```python
from build123d import *

# Parameters (mm, degrees)
ESQUISSE1_R        = 2.5
BOSS_EXTRU_2_DEPTH = 5
CONG_2_R           = 2


with BuildPart() as part:
    # Esquisse1 → Boss.-Extru.2 (new body)
    with BuildSketch(Plane.XY):
        Polygon((-39.751873238, 27.403100775), (30.248126762, 27.403100775), (30.248126762, -27.596899225), (14.016967887, -27.596899225), (-39.751873238, 24.689922481), align=None)
        with Locations((22.936263184, 20.04525616)):
            Circle(ESQUISSE1_R, mode=Mode.SUBTRACT)
        with Locations((22.936263184, -19.519610844)):
            Circle(ESQUISSE1_R, mode=Mode.SUBTRACT)
    extrude(amount=BOSS_EXTRU_2_DEPTH)

    # Congé2
    cong_2_edges = [part.edges().sort_by_distance(p)[0] for p in [
        (-39.751873238, 24.689922481, 2.5),
    ]]
    fillet(cong_2_edges, radius=CONG_2_R)


solid = part.part
```
Geometry: final body of the model. Coordinates: model frame, mm. Give positions to 0.01 mm unless a question says otherwise; leave off trailing zeros. Loops run counter-clockwise (first coordinate to the right, second up) from the corner with the lowest first, then second, coordinate; pieces in that order, holes last. Notation, with made-up numbers: (-25, 39) -> (11, 39) arc R21 cw to (11, 45) -> close; hole circle Ø3 at (35, 27.5). An arc over 180 degrees is marked (long way). Use CSV: the item, a comma, the result in double quotes.
(1) Pull-direction query (X, two-part tool) for faces 1 (the face through (21.09, 21.73, 2.46)), 2 (the face through (-12.2, -2.1, 2.5)), 3 (the face through (30.248, 0, 2)); classes: released by +X, released by -X, zero draft, split by the parting line, or undercut.
From the geometry:
face 1,"undercut"
face 2,"released by -X"
face 3,"released by +X"
(2) Ray query, line 1 along Y through (x, z) = (23.5, 3.85); line 2 along Y through (x, z) = (24.5, 2.6); line 3 along X through (y, z) = (-21.5, 2.95). Return the intervals inside material, ascending. Write a range as [from, to].
From the geometry:
line 1,"[-27.6, -21.96], [-17.08, 17.61], [22.48, 27.4]"
line 2,"[-27.6, -21.47], [-17.57, 18.09], [22, 27.4]"
line 3,"[7.75, 21.41], [24.46, 30.25]"
(3) Cut plane C-C (x = -5). Output: boundary loops of the cut face in (y, z).
From the geometry:
outline,"(-9.1, 0) -> (27.4, 0) -> (27.4, 5) -> (-9.1, 5) -> close"
(4) Cut plane D-D (y = -3.5). Output: boundary loops of the cut face in (x, z).
From the geometry:
outline,"(-10.76, 0) -> (30.25, 0) -> (30.25, 5) -> (-10.76, 5) -> close"
(5) Cut plane A-A (z = 1.95). Output: boundary loops of the cut face in (x, y).
From the geometry:
outline,"(-39.75, 25.53) arc R2 ccw to (-39.15, 24.1) -> (14.02, -27.6) -> (30.25, -27.6) -> (30.25, 27.4) -> (-39.75, 27.4) -> close; hole circle Ø5 at (22.94, -19.52); hole circle Ø5 at (22.94, 20.05)"
(6) First-contact query: P1, Ø1, axis at x = 8, z = 3, coming from the -Y side; P2, Ø4, axis at x = 22.94, y = 20.05, coming from the +Z side (1 decimal). Flat tips, straight axial feed; report the tip coordinate or a pass-through.
From the geometry:
P1,"y = -22.23"
P2,"through"
(7) Cut plane B-B (y = 21). Output: boundary loops of the cut face in (x, z).
From the geometry:
outline,"(-35.96, 0) -> (20.63, 0) -> (20.63, 5) -> (-35.96, 5) -> close; (25.25, 0) -> (30.25, 0) -> (30.25, 5) -> (25.25, 5) -> close"
